Geometry: final body of the model. Coordinates: model frame, mm. Face numbers are marked on the shaded views. A direction names the side the tool comes from. Round coordinates to 2 decimals unless told otherwise and drop trailing zeros. Write each loop counter-clockwise with the first axis right and the second up, starting at its lowest first coordinate (ties: lowest second). Pieces come first, ordered by that corner, then holes. Notation, with made-up numbers: (44, 89.5) - (70, 89.5) arc R23 cw to (70, 97.5) - close; hole circle Ø7 at (-13, 11.5). An arc over 180 degrees is marked (long way). Write each question's results on one line, items separated by ' | '.
from build123d import *

# Parameters (mm, degrees)
SKETCH1_W           = 46
SKETCH1_H           = 50
BOSS_EXTRUDE1_DEPTH = 5
SKETCH2_W           = 30
SKETCH2_H           = 13
BOSS_EXTRUDE2_DEPTH = 12.5
SKETCH3_W           = 46
SKETCH3_H           = 2
BOSS_EXTRUDE3_DEPTH = 22
SKETCH4_R           = 1.75
CUT_EXTRUDE1_DEPTH  = 22
SKETCH5_W           = 15
SKETCH5_H           = 5
SKETCH5_W_2         = 5
CUT_EXTRUDE2_DEPTH  = 2
SKETCH6_R           = 2.4
BOSS_EXTRUDE6_DEPTH = 2
FILLET1_R           = 2


with BuildPart() as part:
    # Sketch1 → Boss-Extrude1 (new body)
    with BuildSketch(Plane(origin=(0, 0, 0), x_dir=(1, 0, 0), z_dir=(0, 1, 0))):
        with Locations((23, 25)):
            Rectangle(SKETCH1_W, SKETCH1_H)
    extrude(amount=BOSS_EXTRUDE1_DEPTH)

    # Sketch2 → Boss-Extrude2 (add)
    with BuildSketch(Plane(origin=(0, 5, 0), x_dir=(1, 0, 0), z_dir=(0, 1, 0))):
        with Locations((23, 14)):
            Rectangle(SKETCH2_W, SKETCH2_H)
    extrude(amount=BOSS_EXTRUDE2_DEPTH)

    # Sketch3 → Boss-Extrude3 (add)
    with BuildSketch(Plane.XZ):
        with Locations((23, -1)):
            Rectangle(SKETCH3_W, SKETCH3_H)
    extrude(amount=BOSS_EXTRUDE3_DEPTH)

    # Sketch4 → Cut-Extrude1 (cut)
    with BuildSketch(Plane(origin=(0, 0, -2), x_dir=(-1, 0, 0), z_dir=(0, 0, -1))):
        with Locations((-23, -17)):
            Circle(SKETCH4_R)
    extrude(amount=-CUT_EXTRUDE1_DEPTH, mode=Mode.SUBTRACT)

    # Sketch5 → Cut-Extrude2 (cut)
    with BuildSketch(Plane(origin=(0, 17.5, 0), x_dir=(1, 0, 0), z_dir=(0, 1, 0))):
        with Locations((16.5, 14)):
            Rectangle(SKETCH5_W, SKETCH5_H)
        with Locations((34.5, 14)):
            Rectangle(SKETCH5_W_2, SKETCH5_H)
        Polygon((31, 17.5), (31, 10.5), (38, 10.5), (38, 7.5), (8, 7.5), (8, 10.5), (25, 10.5), (25, 17.5), (8, 17.5), (8, 20.5), (38, 20.5), (38, 17.5), align=None)
    extrude(amount=-CUT_EXTRUDE2_DEPTH, mode=Mode.SUBTRACT)

    # Sketch6 → Boss-Extrude6 (add)
    with BuildSketch(Plane(origin=(0, 15.5, 0), x_dir=(1, 0, 0), z_dir=(0, 1, 0))):
        with Locations(Location((11.5, 14, 0), (0, 0, 270))):
            Circle(SKETCH6_R)
        with Locations(Location((34.5, 14, 0), (0, 0, 90))):
            Circle(SKETCH6_R)
    extrude(amount=BOSS_EXTRUDE6_DEPTH)

    # Fillet1
    fillet1_edges = [part.edges().sort_by_distance(p)[0] for p in [
        (11.5, 17.5, -16.4),
        (34.5, 17.5, -11.6),
    ]]
    fillet(fillet1_edges, radius=FILLET1_R - 0.0001)  # a hair under: the kernel refuses the full size


solid = part.part
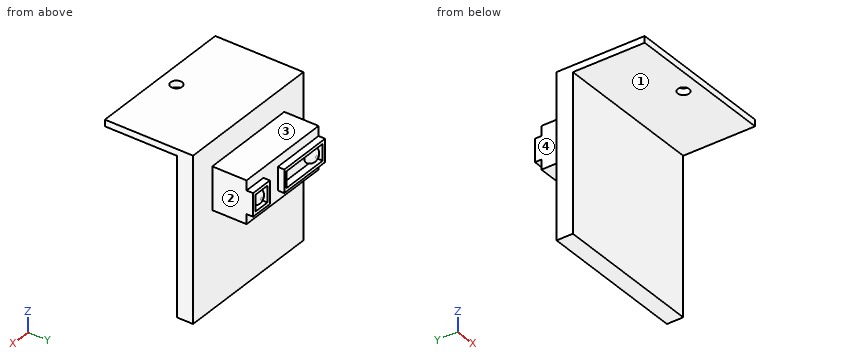
Q1. Section query B-B, the plane y = -17. Return loops of the section in (x, z).
Answer block:
outline: (0, -2) - (21.25, -2) - (21.25, 0) - (0, 0) - close; (24.75, -2) - (46, -2) - (46, 0) - (24.75, 0) - close
Q2. Section query C-C, the plane x = 42.5. Return loops of the section in (y, z).
Answer block:
outline: (-22, -2) - (0, -2) - (0, -50) - (5, -50) - (5, 0) - (-22, 0) - close
Q3. Ray query, line 1 along Y through (x, z) = (23, -1.4); line 2 along Z through (x, y) = (8, -19); line 3 along Y through (x, z) = (32, -6). Return the intervals inside material, ascending.
Answer block:
line 1: -22 to -18.75, -15.25 to 5 | line 2: -2 to 0 | line 3: 0 to 5
Q4. Section query D-D, the plane y = 14. Return loops of the section in (x, z), plus the area to 3 significant figures.
Answer block:
outline: (8, -20.5) - (38, -20.5) - (38, -7.5) - (8, -7.5) - close | area: 390 mm2
Q5. Access query for the marked faces 1, 2, 3 and 4. Directions: +Z, -Z, +X, -X, +Y, -Y. A direction counts if a zero-diameter tool reaches every point of the face in a straight line with its end or side. Return the directions, or none.
Answer block:
face 1: -Z, +X, -X, -Y | face 2: +Z, -Z, +X, +Y | face 3: +Z, +X, -X, +Y | face 4: +Z, -Z, -X, +Y
Q6. Section query A-A, the plane x = 23. Return loops of the section in (y, z).
Answer block:
outline: (-22, -2) - (-18.75, -2) - (-18.75, 0) - (-22, 0) - close; (-15.25, -2) - (0, -2) - (0, -50) - (5, -50) - (5, -20.5) - (15.5, -20.5) - (15.5, -17.5) - (17.5, -17.5) - (17.5, -16.5) - (15.5, -16.5) - (15.5, -11.5) - (17.5, -11.5) - (17.5, -10.5) - (15.5, -10.5) - (15.5, -7.5) - (5, -7.5) - (5, 0) - (-15.25, 0) - close
Q7. Pin query (flat end, axial travel): pin 1 (2 mm diameter, centred on x = 17, y = 17, fed in from -Z); pin 2 (8.5 mm diameter, centred on x = 30, y = 11.5, fed in from +Z); pin 3 (1 mm diameter, centred on x = 34, y = 17, fed in from +Z). Return the tip coordinate at first contact, or that it passes through.
Answer block:
pin 1: z = -17.5 | pin 2: z = -7.5 | pin 3: z = -10.5
